Job drawing, mm, ordinate dimensions from the low corner. One solid piece. A direction names the side the tool comes from. Give positions to 0.01 mm unless a question says otherwise; leave off trailing zeros. Order: outer loops, then holes, each group sorted by start corner. A loop starts at its lowest first (then second) coordinate and runs counter-clockwise, first axis right, second up. Notation, with made-up numbers: (11.25, 2) -> (68.25, 2) arc R16 ccw to (68.25, 7) -> close; hole circle Ø7 at (83, 82). An arc over 180 degrees is marked (long way). Use CSV: the item, a comma, the result in double quotes. Start each with the question number.
1. Wall check: line 1 (Y direction, x = 30, z = 5.25) (1 decimal); line 2 (Y direction, x = 28.5, z = 6.75); line 3 (Z direction, x = 18, y = 2.5) (1 decimal). Give the ranges that are in metal, low to high. Write a range as from..to.
2. Cut at A-A on y = 2.5. List the corners of the cut face in (x, z) (1 decimal).
3. Cut at B-B on z = 6. List the corners of the cut face in (x, y) (1 decimal), then the cut area to 3 significant figures.
4. Drop flat-ended pins along their axis: pin 1 (1 mm diameter, centred on x = 7.5, z = 7.5, fed in from -Y); pin 2 (3 mm diameter, centred on x = 27.5, y = 1.5, fed in from +Z); pin 3 (3 mm diameter, centred on x = 23, z = 2.5, fed in from -Y) (1 decimal). Give the stop position or say it passes through.
5. Cut at C-C on x = 34.5. List the corners of the cut face in (y, z) (1 decimal).
6. 3-axis set-ups, long thin cutter, end or side, ignore diameter. For the marked faces 1 and 2: which of +Z, -Z, +X, -X, +Y, -Y reach the whole face in a straight line?
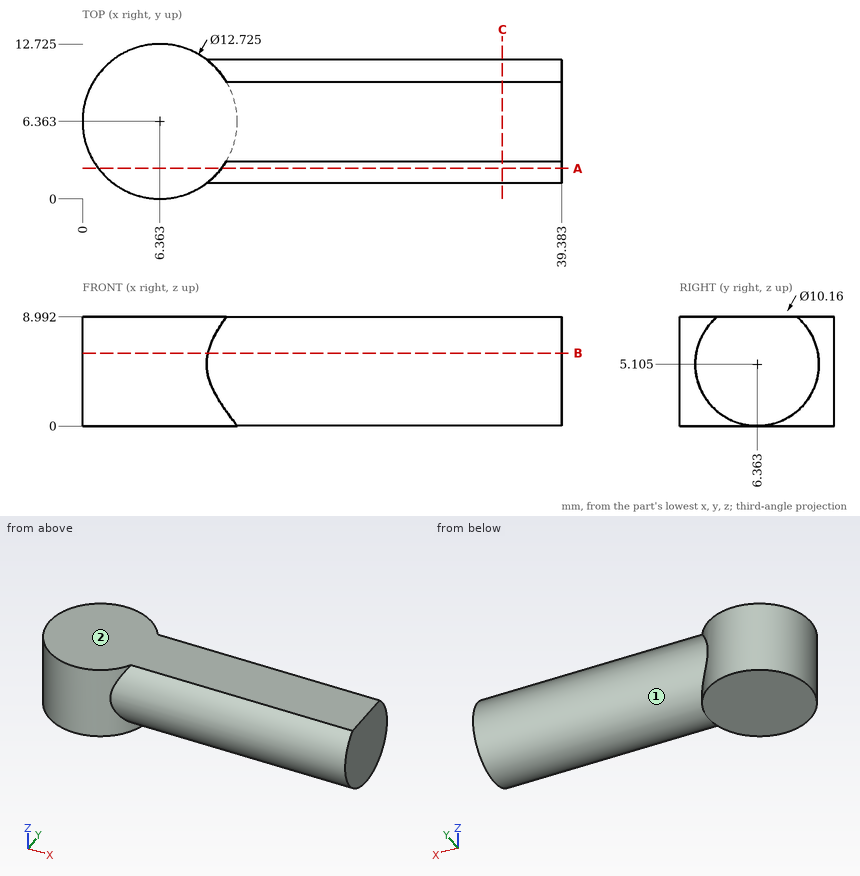
Verdict:
1,line 1,"1.3..11.4"
1,line 2,"1.56..11.17"
1,line 3,"1.8..8.4"
2,outline,"(1.3, 0) -> (11.4, 0) -> (11.4, 1.8) -> (39.4, 1.8) -> (39.4, 8.4) -> (11.4, 8.4) -> (11.4, 9) -> (1.3, 9) -> close"
3,outline,"(10.3, 1.4) -> (39.4, 1.4) -> (39.4, 11.4) -> (10.3, 11.4) arc R6.4 ccw (long way) to start"
3,area,"401 mm^2"
4,pin 1,"y = 0.03"
4,pin 2,"z = 8.91"
4,pin 3,"y = 1.4"
5,outline,"(3.1, 9) arc R5.1 ccw (long way) to (9.6, 9) -> close"
6,face 1,"+X"
6,face 2,"+Z, +X, -X, +Y, -Y"
